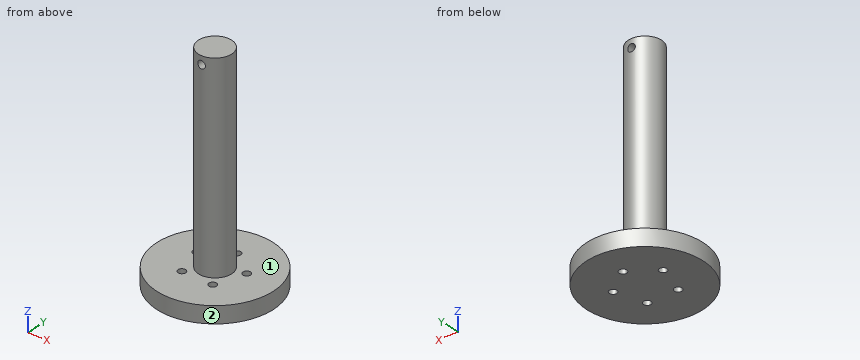
from build123d import *

# Parameters (mm, degrees)
SKETCH1_R           = 44.45
SKETCH1_R_2         = 2.921
BOSS_EXTRUDE1_DEPTH = 12.7
SKETCH2_R           = 12.7
BOSS_EXTRUDE2_DEPTH = 152.4
CUT_EXTRUDE1_REACH  = 182.277
SKETCH4_R           = 2.921


with BuildPart() as part:
    # Sketch1 → Boss-Extrude1 (new body)
    with BuildSketch(Plane.XY):
        Circle(SKETCH1_R)
        with Locations((0, 20.32)):
            Circle(SKETCH1_R_2, mode=Mode.SUBTRACT)
        with Locations((19.325468411, 6.279225326)):
            Circle(SKETCH1_R_2, mode=Mode.SUBTRACT)
        with Locations((11.943796327, -16.439225326)):
            Circle(SKETCH1_R_2, mode=Mode.SUBTRACT)
        with Locations((-11.943796327, -16.439225326)):
            Circle(SKETCH1_R_2, mode=Mode.SUBTRACT)
        with Locations((-19.325468411, 6.279225326)):
            Circle(SKETCH1_R_2, mode=Mode.SUBTRACT)
    extrude(amount=BOSS_EXTRUDE1_DEPTH)

    # Sketch2 → Boss-Extrude2 (add)
    with BuildSketch(Plane.XY.offset(12.7)):
        with Locations(Location((0, 0, 0), (0, 0, 180))):
            Circle(SKETCH2_R)
    extrude(amount=BOSS_EXTRUDE2_DEPTH)

    # Sketch4 → Cut-Extrude1 (cut, up to next)
    with BuildSketch(Plane(origin=(0, -12.7, 0), x_dir=(-1, 0, 0), z_dir=(0, -1, 0)), mode=Mode.PRIVATE) as cut_extrude1_sk1:
        with Locations(Location((0, -158.75, 0), (0, 0, 90))):
            Circle(SKETCH4_R)
    cut_extrude1_tool1 = extrude(cut_extrude1_sk1.sketch, amount=-CUT_EXTRUDE1_REACH, mode=Mode.PRIVATE) & part.part
    add(cut_extrude1_tool1.solids().sort_by_distance((0, -12.7, 158.75))[0], mode=Mode.SUBTRACT)


solid = part.part
Read the model definition and answer for the solid it produces. Units are mm, in the model's axes. Face numbers are marked on the shaded views. A direction names the side the tool comes from. Coordinates: 2 decimals unless noted, no trailing zeros. Loops run counter-clockwise (first coordinate to the right, second up) from the corner with the lowest first, then second, coordinate; pieces in that order, holes last. Notation, with made-up numbers: (-6, 69.5) -> (32, 69.5) arc R5 cw to (32, 74.5) -> close; hole circle Ø10 at (88, -33). An arc over 180 degrees is marked (long way). Write item = value, one per line. Start each with the question number.
1) The part is cut by section A-A, the plane x = 0. Determine the outline of the cut face in (y, z), plus the area to 3 significant figures.
2) For the marked faces 1 and 2, determine the directions among +Z, -Z, +X, -X, +Y, -Y from which every point of the face is accessible in a straight line to the end or side of a thin tool.
3) Find the intervals of material crossed by L1, parallel to Z at x = -31, y = 4; L2, parallel to X at y = -1, z = 32.5; L3, parallel to Z at x = 0.5, y = 5, in increasing order. Write a range as from..to.
4) The part is cut by section D-D, the plane z = 158.75. Determine the outline of the cut face in (x, y).
5) The part is cut by section C-C, the plane z = 79. Determine the outline of the cut face in (x, y).
6) Given P1, Ø6, axis at x = -1, z = 127, coming from the +Y side; P2, Ø7.5, axis at x = 19.33, y = 6.28, coming from the +Z side; P3, Ø6, axis at x = 15.5, y = -26, coming from the -Z side; P4, Ø7.5, axis at x = 0, z = 158.75, coming from the -Y side, each flat-ended and moving along its own axis, determine where each tip first touches the part or whether it passes through.
7) The part is cut by section B-B, the plane y = 20.32. Determine the outline of the cut face in (x, z), plus the area to 3 significant figures.
Result:
q1.outline = (-44.45, 0) -> (17.4, 0) -> (17.4, 12.7) -> (12.7, 12.7) -> (12.7, 155.83) -> (-12.7, 155.83) -> (-12.7, 12.7) -> (-44.45, 12.7) -> close; (-12.7, 161.67) -> (12.7, 161.67) -> (12.7, 165.1) -> (-12.7, 165.1) -> close; (23.24, 0) -> (44.45, 0) -> (44.45, 12.7) -> (23.24, 12.7) -> close
q1.area = 4,780 mm²
q2.face_1 = +Z
q2.face_2 = +Z, -Z
q3.L1 = 0..12.7
q3.L2 = -12.66..12.66
q3.L3 = 0..155.87, 161.63..165.1
q4.outline = (-2.92, -12.36) -> (-2.92, 12.36) arc R12.7 ccw to start; (2.92, -12.36) arc R12.7 ccw to (2.92, 12.36) -> close
q5.outline = circle Ø25.4 at (0, 0)
q6.P1 = 12.7
q6.P2 = 12.7
q6.P3 = 0
q6.P4 = -12.7
q7.outline = (-39.53, 0) -> (-2.92, 0) -> (-2.92, 12.7) -> (-39.53, 12.7) -> close; (2.92, 0) -> (39.53, 0) -> (39.53, 12.7) -> (2.92, 12.7) -> close
q7.area = 930 mm²
